Autodesk Inventor part; units mm, degrees
ref_plane "YZ Plane" through (0, 0, 0) normal (1, 0, 0) x (0, 1, 0)
ref_plane "XZ Plane" through (0, 0, 0) normal (0, 1, 0) x (-1, 0, 0)
ref_plane "XY Plane" through (0, 0, 0) normal (0, 0, 1) x (1, 0, 0)
sketch "草圖1" plane through (0, 0, 0) normal (0, 1, 0) x (-1, 0, 0)
  circle A0 centre (0, 0) radius 1.5
  line L0 (0, 0) -> (-40, 0)
  circle A1 centre (-40, 0) radius 1.5
  line L1 (-40, 0) -> (-41.7431, 19.9239)
  circle A2 centre (-41.7431, 19.9239) radius 1.5
  circle A3 centre (0, 0) radius 4
  circle A4 centre (-40, 0) radius 4
  circle A5 centre (-41.7431, 19.9239) radius 4
  arc A6 (-43.4405, 2.0403) -> (-44.7771, 17.3172) centre (-54.7513, 8.7476) ccw
  arc A7 (-1.3167, -3.7771) -> (-38.6833, -3.7771) centre (-20, -57.374) ccw
  arc A8 (-38.9519, 22.789) -> (0.4722, 3.972) centre (8.4988, 71.4966) ccw
  dimension "d0" = 3
  dimension "d1" = 40
  dimension "d2" = 3
  dimension "d3" = 95
  dimension "d4" = 20
  dimension "d5" = 3
  dimension "d6" = 8
  dimension "d7" = 8
  dimension "d8" = 8
  dimension "d9" = 13.15
  dimension "d10" = 56.76
  dimension "d11" = 68
extrude "擠出1" add sketch "草圖1" along normal mid plane 3 contours A3 | A3 A7 A4 L0 | L0 A4 L1 A5 A8 A3 | A4 L1 A1 L0 | L0 A1 L1 A4 | A4 A6 A5 L1 | A5
properties part number "連接2"
Source: CAD feature listing. Evaluate the final solid. Frame: model axes, mm. Give positions to 0.01 mm unless a question says otherwise; leave off trailing zeros. Write each loop counter-clockwise with the first axis right and the second up, starting at its lowest first coordinate (ties: lowest second). Pieces come first, ordered by that corner, then holes. Notation, with made-up numbers: M 60.5,-39.5 L 87.5,-39.5 A17 cw 87.5,-28.5 Z; hole C 23,19 d5. An arc over 180 degrees is marked long. Return JSON: item names as keys, results as strings. Group by question number.
1) Cut plane B-B, the plane y = 0.9. Output: boundary loops of the cut face in (x, z).
2) Draft query along X for faces 1 (the face through (20.511, -0.021, 9.995)), 2 (the face through (27, -1.5, 7)), 3 (the face through (40.937, -0.021, 18.659)). Return one class per face: released by +X, released by -X, zero draft, split by the parting line, or undercut.
3) Cut plane D-D, the plane x = 41. Output: boundary loops of the cut face in (y, z).
4) Ray query, L1, parallel to X at y = -0.35, z = 0; L2, parallel to X at y = -0.35, z = 19.25; L3, parallel to Z at x = 0, y = 0.05. Return the intervals inside material, ascending.
5) First-contact query: pin 1 Ø1.5 at (x, y) = (9.5, 1) entering from -Z; pin 2 Ø2.5 at (x, z) = (0, 0) entering from +Y; pin 3 Ø1 at (y, z) = (0.5, 1) entering from +X. Flat tips, straight axial feed; report the tip coordinate or a pass-through.
6) Cut plane C-C, the plane x = 0. Output: boundary loops of the cut face in (y, z).
7) Cut plane A-A, the plane z = 0. Output: boundary loops of the cut face in (x, y), then the cut area to 3 significant figures.
Data:
{
 "1": {"outline": "M -0.47,3.97 A4 ccw long 1.32,-3.78 A56.76 cw 38.68,-3.78 A4 ccw 43.44,2.04 A13.15 cw 44.78,17.32 A4 ccw 38.95,22.79 A68 cw Z; hole C 0,0 d3; hole C 40,0 d3; hole C 41.74,19.92 d3"},
 "2": {"face 1": "released by -X", "face 2": "zero draft", "face 3": "undercut"},
 "3": {"outline": "M -1.5,-3.87 L 1.5,-3.87 L 1.5,-1.12 L -1.5,-1.12 Z; M -1.5,1.12 L 1.5,1.12 L 1.5,18.62 L -1.5,18.62 Z; M -1.5,21.23 L 1.5,21.23 L 1.5,23.85 L -1.5,23.85 Z"},
 "4": {"L1": "x = -4 to -1.5, 1.5 to 38.5, 41.5 to 44", "L2": "x = 35.02 to 40.4, 43.08 to 45.69", "L3": "z = -4 to -1.5, 1.5 to 4.03"},
 "5": {"pin 1": "stops at z = -1.74", "pin 2": "passes through", "pin 3": "stops at x = 43.97"},
 "6": {"outline": "M -1.5,-4 L 1.5,-4 L 1.5,-1.5 L -1.5,-1.5 Z; M -1.5,1.5 L 1.5,1.5 L 1.5,4.03 L -1.5,4.03 Z"},
 "7": {"outline": "M -4,-1.5 L -1.5,-1.5 L -1.5,1.5 L -4,1.5 Z; M 1.5,-1.5 L 38.5,-1.5 L 38.5,1.5 L 1.5,1.5 Z; M 41.5,-1.5 L 44,-1.5 L 44,1.5 L 41.5,1.5 Z", "area": "126 mm²"}
}
